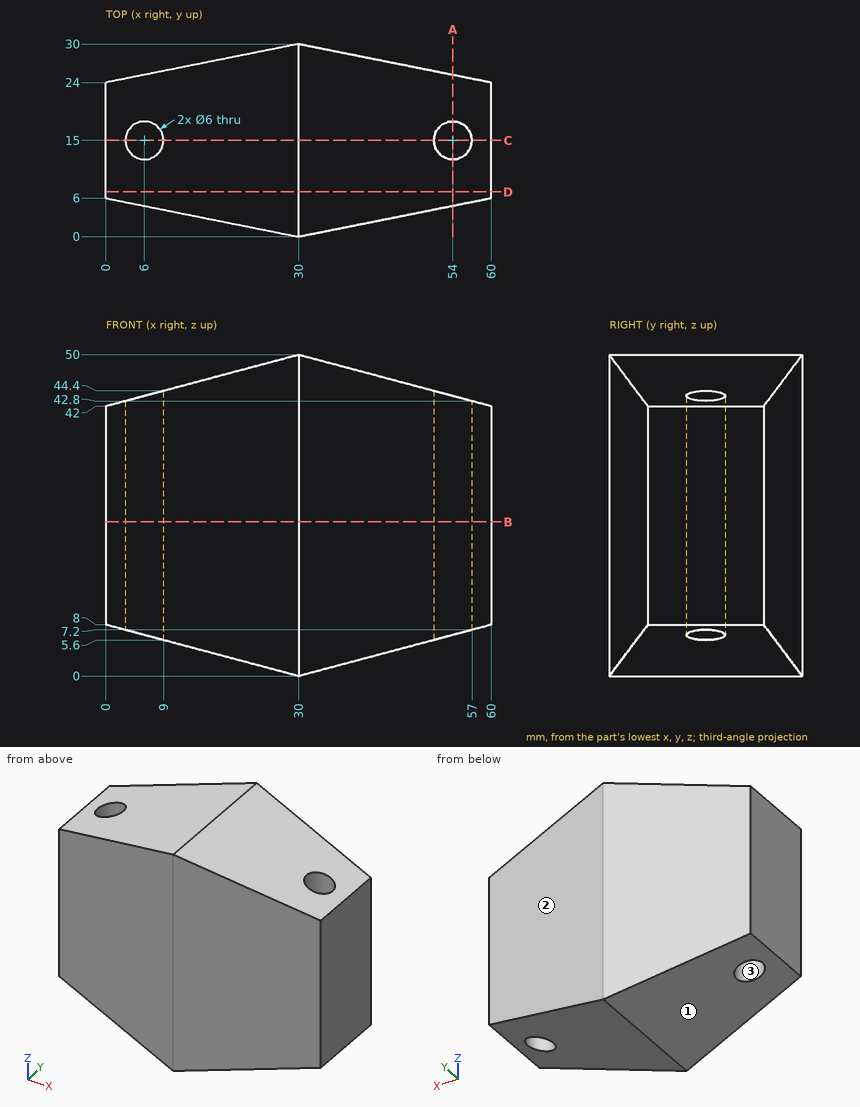
Job drawing, mm, ordinate dimensions from the low corner. One solid piece. Round coordinates to 2 decimals unless told otherwise and drop trailing zeros. Order: outer loops, then holes, each group sorted by start corner. A loop starts at its lowest first (then second) coordinate and runs counter-clockwise, first axis right, second up. Notation, with made-up numbers: (55.25, 22) -> (80.25, 22) arc R11 cw to (80.25, 32) -> close; hole circle Ø1 at (70, 36.5). An arc over 180 degrees is marked (long way). Answer in a Markdown table with one row per item.
1) Band-saw the part on A-A on x = 54. Give the cut face in (y, z).
Values:
| item | result |
|---|---|
| outline | (4.8, 6.4) -> (12, 6.4) -> (12, 43.6) -> (4.8, 43.6) -> close; (18, 6.4) -> (25.2, 6.4) -> (25.2, 43.6) -> (18, 43.6) -> close |
2) Wall check: L1, parallel to X at y = 15, z = 15; L2, parallel to Y at x = 5, z = 40; L3, parallel to Y at x = 6, z = 18.5. Give the ranges that are in metal, low to high.
Values:
| item | result |
|---|---|
| L1 | 0 to 3, 9 to 51, 57 to 60 |
| L2 | 5 to 12.17, 17.83 to 25 |
| L3 | 4.8 to 12, 18 to 25.2 |
3) Band-saw the part on B-B on z = 24. Give the cut face in (x, y), and give its area (3 significant figures).
Values:
| item | result |
|---|---|
| outline | (0, 6) -> (30, 0) -> (60, 6) -> (60, 24) -> (30, 30) -> (0, 24) -> close; hole circle Ø6 at (6, 15); hole circle Ø6 at (54, 15) |
| area | 1,380 mm2 |
4) Pin check, flat tips, straight feed: P1, Ø2, axis at x = 52, z = 5.5, coming from the -Y side; P2, Ø8, axis at x = 43, y = 11, coming from the -Z side; P3, Ø7, axis at x = 54, y = 15, coming from the +Z side. Stop position of each tip, or through.
Values:
| item | result |
|---|---|
| P1 | y = 4.2 |
| P2 | z = 2.4 |
| P3 | z = 44.53 |
5) Band-saw the part on D-D on y = 7. Give the cut face in (x, z), and give its area (3 significant figures).
Values:
| item | result |
|---|---|
| outline | (0, 8) -> (30, 0) -> (60, 8) -> (60, 42) -> (30, 50) -> (0, 42) -> close |
| area | 2,520 mm2 |
6) Mould opens along Y. For the marked faces 1, 2 and 3 say: released by +Y, released by -Y, zero draft, split by the parting line, or undercut.
Values:
| item | result |
|---|---|
| face 1 | zero draft |
| face 2 | released by +Y |
| face 3 | undercut |
7) Band-saw the part on C-C on y = 15. Give the cut face in (x, z), and give its area (3 significant figures).
Values:
| item | result |
|---|---|
| outline | (0, 8) -> (3, 7.2) -> (3, 42.8) -> (0, 42) -> close; (9, 5.6) -> (30, 0) -> (51, 5.6) -> (51, 44.4) -> (30, 50) -> (9, 44.4) -> close; (57, 7.2) -> (60, 8) -> (60, 42) -> (57, 42.8) -> close |
| area | 2,070 mm2 |
